```python
from build123d import *

# Parameters (mm, degrees)
EXTRUDE_THIN1_DEPTH   = 3
SKETCH1_3_R           = 3
BOSS_EXTRUDE1_DEPTH   = 3
FILLET1_R             = 5
F_2_5MM_DOWEL_HOLE1_D = 2.5
CHAMFER1_SIZE         = 0.25


with BuildPart() as part:
    # Sketch1 → Extrude-Thin1 (new body)
    with BuildSketch(Plane.XY):
        with BuildLine():
            ThreePointArc((67.932775445, 34.102173105), (58.457726976, 34.411419672), (50.491619232, 29.272032126))
            ThreePointArc((50.491619232, 29.272032126), (42.436789288, 23.388051771), (32.560988498, 21.984460302))
            Line((32.560988498, 21.984460302), (18.0194176, 23.497567077))
            ThreePointArc((18.0194176, 23.497567077), (10.297542455, 21.776854665), (5.1667157, 15.754992513))
            Line((5.1667157, 15.754992513), (-0.737799909, 1.088733357))
            Line((-0.737799909, 1.088733357), (2.04513605, -0.031653828))
            Line((2.04513605, -0.031653828), (7.949651659, 14.634605328))
            ThreePointArc((7.949651659, 14.634605328), (11.845577871, 19.207110251), (17.7089323, 20.513677186))
            Line((17.7089323, 20.513677186), (32.250503198, 19.000570412))
            ThreePointArc((32.250503198, 19.000570412), (43.566353212, 20.608827896), (52.795705795, 27.350786407))
            ThreePointArc((52.795705795, 27.350786407), (59.258407694, 31.520241644), (66.94527507, 31.269357719))
            Line((66.94527507, 31.269357719), (67.932775445, 34.102173105))
        make_face()
    extrude(amount=EXTRUDE_THIN1_DEPTH)

    # Sketch1<3> → Boss-Extrude1 (add, through all)
    with BuildSketch(Plane.XY):
        with Locations((0.653668071, 0.528539764)):
            Circle(SKETCH1_3_R)
        with Locations((67.439025258, 32.685765412)):
            Circle(SKETCH1_3_R)
    extrude(amount=BOSS_EXTRUDE1_DEPTH)

    # Fillet1
    fillet1_edges = [part.edges().sort_by_distance(p)[0] for p in [
        (0.232483855, 3.498826595, 1.5),
        (3.015419815, 2.37843941, 1.5),
        (64.556717413, 31.853718847, 1.5),
        (65.287195047, 34.77613063, 1.5),
    ]]
    fillet(fillet1_edges, radius=FILLET1_R)

    # Ø2.5mm Dowel Hole1 (through all)
    with Locations(Plane.XY.offset(3)):
        with Locations((67.439025258, 32.685765412), (0.653668071, 0.528539764)):
            Hole(F_2_5MM_DOWEL_HOLE1_D / 2)

    # Chamfer1
    chamfer1_edges = [part.edges().sort_by_distance(p)[0] for p in [
        (10.297542455, 21.776854665, 0),
        (25.290203049, 22.741013689, 0),
        (42.436789288, 23.388051771, 0),
        (43.566353212, 20.608827896, 0),
        (24.979717749, 19.757123799, 0),
        (5.868250185, 9.464600631, 3),
        (11.845577871, 19.207110251, 0),
        (5.868250185, 9.464600631, 0),
        (3.085314225, 10.584987816, 0),
        (11.845577871, 19.207110251, 3),
        (24.979717749, 19.757123799, 3),
        (43.566353212, 20.608827896, 3),
        (42.436789288, 23.388051771, 3),
        (25.290203049, 22.741013689, 3),
        (10.297542455, 21.776854665, 3),
        (3.085314225, 10.584987816, 3),
        (56.623528898, 30.466570313, 0),
        (56.623528898, 30.466570313, 3),
        (70.396803241, 32.184218401, 0),
        (70.396803241, 32.184218401, 3),
        (56.436616897, 33.701943285, 0),
        (56.436616897, 33.701943285, 3),
        (-0.466719115, -2.254396195, 3),
        (-0.466719115, -2.254396195, 0),
        (63.499669001, 31.670454016, 3),
        (63.499669001, 31.670454016, 0),
        (64.988861472, 35.027622491, 3),
        (64.988861472, 35.027622491, 0),
        (3.437869945, 2.784750939, 0),
        (3.437869945, 2.784750939, 3),
        (0.209401135, 4.084505995, 0),
        (0.209401135, 4.084505995, 3),
    ]]
    chamfer(chamfer1_edges, length=CHAMFER1_SIZE - 0.0001)  # a hair under: the kernel refuses the full size


solid = part.part
```
The model under review builds one solid part; all positions refer to its coordinate system, in mm. A direction names the side the tool comes from. Coordinates: 2 decimals unless noted, no trailing zeros. Order: outer loops, then holes, each group sorted by start corner. A loop starts at its lowest first (then second) coordinate and runs counter-clockwise, first axis right, second up. Notation, with made-up numbers: (73.5, -17.5) -> (93.5, -17.5) arc R20 cw to (93.5, -4.5) -> close; hole circle Ø10 at (36.25, -39.5). An arc over 180 degrees is marked (long way). Answer in a Markdown table with one row per item. Add a question column.
Item 1: To check wall thickness, follow probe 1 along Y at (x, z) = (1, 2.45); probe 2 along X at (y, z) = (31, 1.75); probe 3 along X at (y, z) = (33, 0.4). State the ranges of each line that lie inside material, in increasing order.
Item 2: We need section B-B on y = 10.5. Write out the cut boundary in (x, z), plus the area to 3 significant figures.
Item 3: Clearance check with flat-ended pins moving along their axes: pin 1 (1.5 mm diameter, centred on x = 56, z = 2, fed in from +Y); pin 2 (2 mm diameter, centred on x = 0.65, y = 0.53, fed in from +Z); pin 3 (1 mm diameter, centred on y = 8.5, z = 0.5, fed in from +X); pin 4 (1 mm diameter, centred on x = 60.5, z = 2, fed in from -Y). State where each tip first meets the part, or that it passes through.
Item 4: We need section A-A on x = 31.5. Write out the cut boundary in (y, z), plus the area to 3 significant figures.
Item 5: Machinability: for faces 1 (the cylindrical face through (56.562, 30.434, 1.482)), 2 (the flat face through (25.39, 22.73, 1.48)), 3 (the flat face through (25.38, 22.61, 2.87)), 4 (the flat face through (31, 21, 3)), 5 (the flat face through (24.891, 19.89, 2.873)), which of the approach directions +Z, -Z, +X, -X, +Y, -Y give a long, thin tool a straight path to every point of the face, cutting with its end or side? Answer none if there is none.
Item 6: We need section C-C on z = 1.95. Give the number of separate pieces and of enclosed holes in the cut face, plus the area to 3 significant figures.
Item 7: Mouldability with a two-part tool opening along X and no side actions: class faces 6 (the conical face through (70.259, 32.119, 2.873)), 7 (the cylindrical face through (-0.55, -2.22, 1.48)), 8 (the flat face through (3.229, 10.611, 2.873)) as +X half, -X half, draft (parallel to the pull), parting line (faces both ways), or undercut.
Final values:
| question | item | result |
|---|---|---|
| 1 | probe 1 | y = -2.45 to -0.67, 1.73 to 5.41 |
| 1 | probe 2 | x = 52.17 to 57.75, 64.79 to 69.92 |
| 1 | probe 3 | x = 55 to 66.23, 68.65 to 70.42 |
| 2 | outline | (3.05, 0.25) -> (3.32, 0) -> (6.02, 0) -> (6.29, 0.25) -> (6.29, 2.75) -> (6.02, 3) -> (3.32, 3) -> (3.05, 2.75) -> close |
| 2 | area | 9.57 mm2 |
| 3 | pin 1 | stops at y = 33.83 |
| 3 | pin 2 | passes through |
| 3 | pin 3 | stops at x = 5.68 |
| 3 | pin 4 | stops at y = 31.7 |
| 4 | outline | (19.08, 0.25) -> (19.33, 0) -> (21.84, 0) -> (22.09, 0.25) -> (22.09, 2.75) -> (21.84, 3) -> (19.33, 3) -> (19.08, 2.75) -> close |
| 4 | area | 8.92 mm2 |
| 5 | face 1 | +Z, -Z, -Y |
| 5 | face 2 | +Z, -Z, +Y |
| 5 | face 3 | +Z, +Y |
| 5 | face 4 | +Z, +X, -X, +Y, -Y |
| 5 | face 5 | +Z, -Y |
| 6 | separate pieces | 1 |
| 6 | enclosed holes | 2 |
| 6 | area | 282 mm2 |
| 7 | face 6 | undercut |
| 7 | face 7 | parting line |
| 7 | face 8 | -X half |
